Autodesk Inventor part; units mm, degrees
ref_plane "YZ Plane" through (0, 0, 0) normal (1, 0, 0) x (0, 1, 0)
ref_plane "XZ Plane" through (0, 0, 0) normal (0, 1, 0) x (-1, 0, 0)
ref_plane "XY Plane" through (0, 0, 0) normal (0, 0, 1) x (1, 0, 0)
sketch "Sketch1" plane through (0, 0, 0) normal (0, 1, 0) x (-1, 0, 0)
  line L0 (0, 0) -> (361.95, 0)
  line L1 (361.95, 0) -> (361.95, -312.7502)
  line L2 (361.95, -312.7502) -> (0, -312.7502)
  line L3 (0, -312.7502) -> (0, 0)
  dimension "d0" = 361.95
  dimension "d1" = 312.7502
extrude "Extrusion1" add sketch "Sketch1" along normal blind 12.7
shell "Shell1" thickness 1.5875 removed faces 1 at (-120.65, 0, -104.2501)
sketch "Sketch2" plane through (0, 0, 0) normal (1, 0, 0) x (0, 0, -1)
  line L0 (0, 0) -> (0, -3.175)
  arc A0 (0, -1.5875) -> (1.5875, -3.175) centre (0, -3.175) ccw
  line L1 (1.5875, -3.175) -> (1.5875, 0)
  line L2 (312.7502, 0) -> (0, 0)
  line L3 (1.5875, 0) -> (0, 0)
  dimension "d5" = 3.175
  dimension "d6" = 3.175
extrude "Extrusion2" add sketch "Sketch2" against normal up to surface (361.95 mm away)
sketch "Sketch3" plane through (0, 12.7, 0) normal (0, 1, 0) x (1, 0, 0)
  line L0 (-361.95, 312.7502) -> (-361.95, 0) construction
  line L1 (-361.95, 0) -> (-311.15, 0) construction
  line L2 (-311.15, 0) -> (-311.15, 50.8) construction
  line L3 (-311.15, 50.8) -> (-361.95, 50.8) construction
  line L4 (-361.95, 50.8) -> (-361.95, 0) construction
  circle A0 centre (-311.15, 50.8) radius 20.6375
  point P0 (0, 0)
  dimension "d9" = 50.8
  dimension "d10" = 50.8
  dimension "d11" = 41.275
extrude "Extrusion3" cut sketch "Sketch3" against normal blind 12.7
sketch "Sketch4" plane through (0, 12.7, 0) normal (0, 1, 0) x (1, 0, 0)
  circle A0 centre (-311.15, 50.8) radius 20.6375 construction
  line L0 (-311.15, 50.8) -> (-295.0845, 50.8) construction
  line L1 (-295.0845, 50.8) -> (-295.0845, 66.8655) construction
  line L2 (-295.0845, 66.8655) -> (-311.15, 66.8655) construction
  line L3 (-311.15, 66.8655) -> (-311.15, 50.8) construction
  line L4 (-311.15, 50.8) -> (-327.2155, 50.8) construction
  line L5 (-327.2155, 50.8) -> (-327.2155, 34.7345) construction
  line L6 (-327.2155, 34.7345) -> (-311.15, 34.7345) construction
  line L7 (-311.15, 34.7345) -> (-311.15, 50.8) construction
  line L8 (-295.0845, 66.8655) -> (-327.2155, 66.8655)
  line L9 (-327.2155, 66.8655) -> (-327.2155, 34.7345)
  line L10 (-327.2155, 34.7345) -> (-295.0845, 34.7345)
  line L11 (-295.0845, 34.7345) -> (-295.0845, 66.8655)
  point P0 (0, 0)
  dimension "d14" = 16.0655
  dimension "d15" = 16.0655
  dimension "d16" = 16.0655
  dimension "d17" = 16.0655
hole "Hole1" at (-327.2155, 12.7, -66.8655) at (-295.0845, 12.7, -66.8655) at (-295.0845, 12.7, -34.7345) at (-327.2155, 12.7, -34.7345) direction (0, -1, 0) diameter 3.175 depth 25.4 tip angle 118
equation "\"d15\" = d14"
equation "\"d16\" = d14"
equation "\"d17\" = d14"
properties part number "lid" material "Steel"
Verification items for the finished model (mm, model axes). A direction names the side the tool comes from. Round coordinates to 2 decimals unless told otherwise and drop trailing zeros. Write each loop counter-clockwise with the first axis right and the second up, starting at its lowest first coordinate (ties: lowest second). Pieces come first, ordered by that corner, then holes.
(1) Section check C-C (x = -179.5). Enter the section's corners in (y, z) (1 decimal), plus the area to 3 significant figures.
Returned:
outline: (-3.2, -1.6) - (11.1, -1.6) - (11.1, -311.2) - (0, -311.2) - (0, -312.8) - (12.7, -312.8) - (12.7, 0) - (-1.6, 0) arc R1.6 ccw (long way) to start
area: 543 mm2
(2) Material ranges on line 1 (X direction, y = 8.5, z = -105); line 2 (Z direction, x = -51.5, y = 9.5); line 3 (Z direction, x = -311.15, y = 11.55), recorded low to high.
Returned:
line 1: x = -361.95 to -360.36, -1.59 to 0
line 2: z = -312.75 to -311.16, -1.59 to 0
line 3: z = -312.75 to -71.44, -30.16 to 0
(3) Depth check by flat-ended pin: pin 1 Ø1.5 at (x, y) = (-56.5, 0) entering from +Z; pin 2 Ø2 at (x, z) = (-48, -105) entering from -Y; pin 3 Ø1.5 at (y, z) = (6, -258) entering from +X. Enter the tip coordinate at first touch or a pass-through.
Returned:
pin 1: stops at z = 0
pin 2: stops at y = 11.11
pin 3: stops at x = 0
(4) Section check B-B (x = -311.15). Enter the section's corners in (y, z) (1 decimal).
Returned:
outline: (-3.2, -1.6) - (11.1, -1.6) - (11.1, -30.2) - (12.7, -30.2) - (12.7, 0) - (-1.6, 0) arc R1.6 ccw (long way) to start; (0, -312.8) - (12.7, -312.8) - (12.7, -71.4) - (11.1, -71.4) - (11.1, -311.2) - (0, -311.2) - close
(5) Mould release check, pull along X, two halves, no side actions. Record for faces 4 (the flat face through (-178, 11.112, -154)), 5 (the flat face through (-184, 6, -312.75)), 6 (the flat face through (0, 8, -158)): pulls with the +X half, pulls with the -X half, needs draft (parallel to the pull), parting line crosses it, or undercut.
Returned:
face 4: undercut
face 5: needs draft
face 6: pulls with the +X half
(6) Section check A-A (z = -50.8). Enter the section's corners in (x, y).
Returned:
outline: (-361.95, 0) - (-360.36, 0) - (-360.36, 11.11) - (-331.79, 11.11) - (-331.79, 12.7) - (-361.95, 12.7) - close; (-290.51, 11.11) - (-1.59, 11.11) - (-1.59, 0) - (0, 0) - (0, 12.7) - (-290.51, 12.7) - close
(7) Access from +Z, -Z, +X, -X, +Y, -Y to the whole of each face (thin tool, end or side, straight path). Record for faces 1 (the flat face through (-178, 12.7, -154)), 2 (the flat face through (-1.588, 5, -159)), 3 (the flat face through (-178, 5, 0)).
Returned:
face 1: +Z, -Z, +X, -X, +Y
face 2: -Y
face 3: +Z, +X, -X, +Y
